The model under review builds one solid part; all positions refer to its coordinate system, in mm. Face numbers are marked on the shaded views. Coordinates: 2 decimals unless noted, no trailing zeros. Order: outer loops, then holes, each group sorted by start corner. A loop starts at its lowest first (then second) coordinate and runs counter-clockwise, first axis right, second up. Notation, with made-up numbers: M 69,72 L 121,72 A29 ccw 121,108 Z; hole C -3,75.25 d5. An arc over 180 degrees is marked long. Write each question's results on one line, items separated by ' | '.
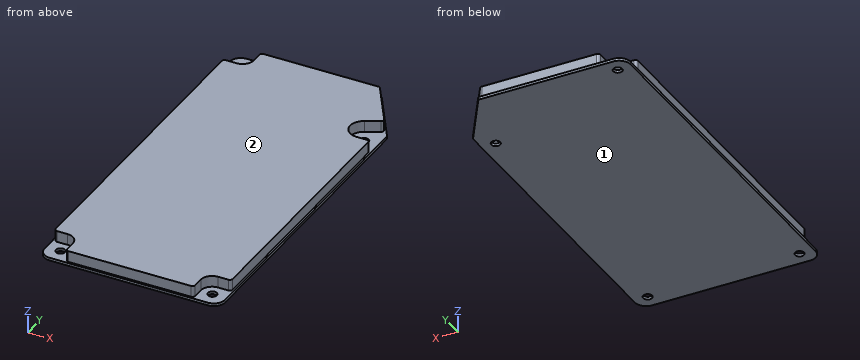
from build123d import *

# Parameters (mm, degrees)
F0_R     = 2.54
F1_DEPTH = 1.5875
F3_DEPTH = 6.35


with BuildPart() as f1:
    # F0 (on Top) → F1 (new body)
    with BuildSketch(Plane.XY):
        with BuildLine():
            ThreePointArc((0, 6.35), (1.859872, 1.859872), (6.35, 0))
            Line((6.35, 0), (95.65005, 0))
            ThreePointArc((95.65005, 0), (100.140178, 1.859872), (102.00005, 6.35))
            Line((102.00005, 6.35), (102.00005, 178.805276))
            ThreePointArc((102.00005, 178.805276), (101.980273, 178.945639), (101.922484, 179.075074))
            Line((101.922484, 179.075074), (82.699306, 209.743598))
            ThreePointArc((82.699306, 209.743598), (82.514847, 209.918278), (82.268873, 209.9818))
            Line((82.268873, 209.9818), (6.35, 209.9818))
            ThreePointArc((6.35, 209.9818), (1.859872, 208.121928), (0, 203.6318))
            Line((0, 203.6318), (0, 6.35))
        make_face()
        with Locations((8.1026, 8.1026)):
            Circle(F0_R, mode=Mode.SUBTRACT)
        with Locations((93.89745, 8.1026)):
            Circle(F0_R, mode=Mode.SUBTRACT)
        with Locations((8.1026, 201.8792)):
            Circle(F0_R, mode=Mode.SUBTRACT)
        with Locations((93.89745, 169.926)):
            Circle(F0_R, mode=Mode.SUBTRACT)
    extrude(amount=F1_DEPTH)

    # F2 (on face) → F3 (join)
    with BuildSketch(Plane.XY.offset(1.5875)):
        with BuildLine():
            Line((81.1149, 208.9912), (16.4465, 208.9912))
            ThreePointArc((16.4465, 208.9912), (15.323968, 208.526232), (14.859, 207.4037))
            Line((14.859, 207.4037), (14.859, 201.46264))
            ThreePointArc((14.859, 201.46264), (12.999128, 196.972512), (8.509, 195.11264))
            Line((8.509, 195.11264), (2.5781, 195.11264))
            ThreePointArc((2.5781, 195.11264), (1.455568, 194.647672), (0.9906, 193.52514))
            Line((0.9906, 193.52514), (0.9906, 16.4465))
            ThreePointArc((0.9906, 16.4465), (1.455568, 15.323968), (2.5781, 14.859))
            Line((2.5781, 14.859), (8.509, 14.859))
            ThreePointArc((8.509, 14.859), (12.999128, 12.999128), (14.859, 8.509))
            Line((14.859, 8.509), (14.859, 2.5781))
            ThreePointArc((14.859, 2.5781), (15.323968, 1.455568), (16.4465, 0.9906))
            Line((16.4465, 0.9906), (85.55355, 0.9906))
            ThreePointArc((85.55355, 0.9906), (86.676082, 1.455568), (87.14105, 2.5781))
            Line((87.14105, 2.5781), (87.14105, 8.509))
            ThreePointArc((87.14105, 8.509), (89.000922, 12.999128), (93.49105, 14.859))
            Line((93.49105, 14.859), (99.325214, 14.859))
            ThreePointArc((99.325214, 14.859), (100.447746, 15.323968), (100.912714, 16.4465))
            Line((100.912714, 16.4465), (100.912714, 160.8709))
            ThreePointArc((100.912714, 160.8709), (100.447746, 161.993432), (99.325214, 162.4584))
            Line((99.325214, 162.4584), (93.622914, 162.4584))
            ThreePointArc((93.622914, 162.4584), (85.981627, 168.480706), (90.051433, 177.317794))
            Line((90.051433, 177.317794), (97.443973, 181.089289))
            ThreePointArc((97.443973, 181.089289), (98.2527, 182.080608), (98.067638, 183.346508))
            Line((98.067638, 183.346508), (82.460005, 208.246818))
            ThreePointArc((82.460005, 208.246818), (81.88357, 208.792694), (81.1149, 208.9912))
        make_face()
    extrude(amount=F3_DEPTH)


solid = f1.part
1) Take a section at B-B on y = 25.5. State the section outline as (x, z) points.
Solutions:
outline: M 0,0 L 102,0 L 102,1.59 L 100.91,1.59 L 100.91,7.94 L 0.99,7.94 L 0.99,1.59 L 0,1.59 Z
2) For pin 1 (4.5 mm diameter, centred on x = 8.1, y = 201.88, fed in from -Z); pin 2 (4.5 mm diameter, centred on y = 4, z = 5.5, fed in from +X); pin 3 (3 mm diameter, centred on x = 6, z = 4.5, fed in from -Y); pin 4 (6.5 mm diameter, centred on x = 8.1, y = 8.1, fed in from +Z), all flat-tipped, find the tip position at first contact; note any pin that passes through.
Solutions:
pin 1: through | pin 2: x = 87.14 | pin 3: y = 14.86 | pin 4: z = 1.59
3) The part is to be moulded in two halves that separate along Z. For the marked faces 1 and 2, say which applies: pulls with the +Z half, pulls with the -Z half, needs draft (parallel to the pull), parting line crosses it, or undercut.
Solutions:
face 1: pulls with the -Z half | face 2: pulls with the +Z half
4) To check wall thickness, follow line 1 along X through (y, z) = (119, 2.25); line 2 along Y through (x, z) = (58, 1.75); line 3 along Y through (x, z) = (92.5, 5.5). State the ranges of each line that lie inside material, in increasing order.
Solutions:
line 1: 0.99 to 100.91 | line 2: 0.99 to 208.99 | line 3: 14.78 to 162.54, 178.57 to 192.23
